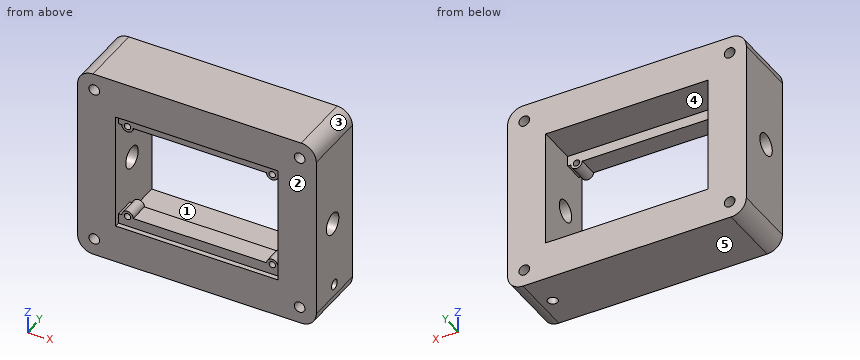
```python
from build123d import *

# Parameters (mm, degrees)
SKETCH1_W               = 94
SKETCH1_H               = 76
SKETCH1_R               = 1.25
BOSS_EXTRUDE1_DEPTH     = 9.8
SKETCH2_W               = 94
SKETCH2_H               = 76
SKETCH2_W_2             = 64
SKETCH2_H_2             = 46
BOSS_EXTRUDE3_DEPTH     = 15.2
SKETCH3_W               = 64
SKETCH3_H               = 46
CUT_EXTRUDE1_DEPTH      = 2
CUT_EXTRUDE2_DEPTH      = 105.427008001
CUT_EXTRUDE2_DEPTH_BACK = 105.427008001
SKETCH4_R               = 4.305
CUT_EXTRUDE3_DEPTH      = 66.406421703
CUT_EXTRUDE3_DEPTH_BACK = 66.406421703
SKETCH5_R               = 2.1
FILLET1_R               = 6
CUT_SWEEP_PROFILE_R     = 1.95


with BuildPart() as part:
    # Sketch1 → Boss-Extrude1 (new body)
    with BuildSketch(Plane(origin=(0, 0, 0), x_dir=(1, 0, 0), z_dir=(0, 1, 0))):
        Rectangle(SKETCH1_W, SKETCH1_H)
        with BuildLine():
            Line((-32, 19), (-30.75, 19))
            ThreePointArc((-30.75, 19), (-28.5, 16.75), (-26.25, 19))
            Line((-26.25, 19), (26.25, 19))
            ThreePointArc((26.25, 19), (28.5, 16.75), (30.75, 19))
            Line((30.75, 19), (32, 19))
            Line((32, 19), (32, -19))
            Line((32, -19), (30.75, -19))
            ThreePointArc((30.75, -19), (28.5, -16.75), (26.25, -19))
            Line((26.25, -19), (-26.25, -19))
            ThreePointArc((-26.25, -19), (-28.5, -16.75), (-30.75, -19))
            Line((-30.75, -19), (-32, -19))
            Line((-32, -19), (-32, 19))
        make_face(mode=Mode.SUBTRACT)
        with Locations(Location((-28.5, 19, 0), (0, 0, 270))):
            Circle(SKETCH1_R, mode=Mode.SUBTRACT)
        with Locations(Location((28.5, 19, 0), (0, 0, 270))):
            Circle(SKETCH1_R, mode=Mode.SUBTRACT)
        with Locations(Location((28.5, -19, 0), (0, 0, 270))):
            Circle(SKETCH1_R, mode=Mode.SUBTRACT)
        with Locations(Location((-28.5, -19, 0), (0, 0, 270))):
            Circle(SKETCH1_R, mode=Mode.SUBTRACT)
    extrude(amount=BOSS_EXTRUDE1_DEPTH)

    # Sketch2 → Boss-Extrude3 (add)
    with BuildSketch(Plane(origin=(0, 9.8, 0), x_dir=(1, 0, 0), z_dir=(0, 1, 0))):
        Rectangle(SKETCH2_W, SKETCH2_H)
        Rectangle(SKETCH2_W_2, SKETCH2_H_2, mode=Mode.SUBTRACT)
    extrude(amount=BOSS_EXTRUDE3_DEPTH)

    # Sketch3 → Cut-Extrude1 (cut)
    with BuildSketch(Plane.XZ):
        Rectangle(SKETCH3_W, SKETCH3_H)
    extrude(amount=-CUT_EXTRUDE1_DEPTH, mode=Mode.SUBTRACT)

    # Sketch4 → Cut-Extrude2 (cut, two sides: drawn at the far end of the back side and taken through both)
    with BuildSketch(Plane(origin=(47, 0, 0), x_dir=(0, 0, -1), z_dir=(1, 0, 0)).offset(-CUT_EXTRUDE2_DEPTH_BACK)):
        with Locations((1, 11.3)):
            Circle(SKETCH4_R)
    extrude(amount=CUT_EXTRUDE2_DEPTH + CUT_EXTRUDE2_DEPTH_BACK, mode=Mode.SUBTRACT)

    # Sketch5 → Cut-Extrude3 (cut, two sides: drawn at the far end of the back side and taken through both)
    with BuildSketch(Plane(origin=(0, 25, 0), x_dir=(1, 0, 0), z_dir=(0, 1, 0)).offset(-CUT_EXTRUDE3_DEPTH_BACK)):
        with Locations(Location((-40.44, 31.44, 0), (0, 0, 270))):
            Circle(SKETCH5_R)
        with Locations(Location((40.44, 31.44, 0), (0, 0, 270))):
            Circle(SKETCH5_R)
        with Locations(Location((40.44, -31.44, 0), (0, 0, 270))):
            Circle(SKETCH5_R)
        with Locations(Location((-40.44, -31.44, 0), (0, 0, 270))):
            Circle(SKETCH5_R)
    extrude(amount=CUT_EXTRUDE3_DEPTH + CUT_EXTRUDE3_DEPTH_BACK, mode=Mode.SUBTRACT)

    # Fillet1
    fillet1_edges = [part.edges().sort_by_distance(p)[0] for p in [
        (-47, 12.5, 38),
        (-47, 12.5, -38),
        (47, 12.5, -38),
        (47, 12.5, 38),
    ]]
    fillet(fillet1_edges, radius=FILLET1_R)

    # Cut-Sweep: sweep along a path in Sketch9
    with BuildLine(Plane(origin=(0, 12.5, 0), x_dir=(-1, 0, 0), z_dir=(0, -1, 0))) as cut_sweep_path:
        Line((-47, 27.34), (-40.44, 27.34))
        ThreePointArc((-40.44, 27.34), (-37.540862197, 28.540862197), (-36.34, 31.44))
        Line((-36.34, 31.44), (-36.34, 38))
    # Cut-Sweep profile (on start of the path) → Cut-Sweep (sweep, cut)
    with BuildSketch(Plane(origin=(47, 12.5, -27.34), x_dir=(0, 0, -1), z_dir=(-1, 0, 0))):
        Circle(CUT_SWEEP_PROFILE_R)
    sweep(path=cut_sweep_path.line, mode=Mode.SUBTRACT)


solid = part.part
```
Geometry: final body of the model. Coordinates: model frame, mm. Face numbers are marked on the shaded views. A direction names the side the tool comes from. Round coordinates to 2 decimals unless told otherwise and drop trailing zeros. Loops run counter-clockwise (first coordinate to the right, second up) from the corner with the lowest first, then second, coordinate; pieces in that order, holes last. Notation, with made-up numbers: (31, 81.25) -> (89, 81.25) arc R28 cw to (89, 108.25) -> close; hole circle Ø3 at (69.5, 80.5). An arc over 180 degrees is marked (long way). Write each question's results on one line, items separated by ' | '.
Item 1: Pull-direction query (X, two-part tool) for the marked faces 1, 2 and 3; classes: pulls with the +X half, pulls with the -X half, needs draft (parallel to the pull), parting line crosses it, or undercut.
Answers below:
face 1: undercut | face 2: needs draft | face 3: pulls with the +X half
Item 2: Cut plane C-C on x = 3. Return the cut outline in (y, z), and give its area (3 significant figures).
Answers below:
outline: (0, -38) -> (25, -38) -> (25, -23) -> (9.8, -23) -> (9.8, -19) -> (2, -19) -> (2, -23) -> (0, -23) -> close; (0, 23) -> (2, 23) -> (2, 19) -> (9.8, 19) -> (9.8, 23) -> (25, 23) -> (25, 38) -> (0, 38) -> close | area: 812 mm²
Item 3: Cut plane B-B on x = -28.5. Return the cut outline in (y, z), and give its area (4 significant figures).
Answers below:
outline: (0, -38) -> (25, -38) -> (25, -23) -> (9.8, -23) -> (9.8, -20.25) -> (2, -20.25) -> (2, -23) -> (0, -23) -> close; (0, 23) -> (2, 23) -> (2, 20.25) -> (9.8, 20.25) -> (9.8, 23) -> (25, 23) -> (25, 38) -> (0, 38) -> close; (2, -17.75) -> (9.8, -17.75) -> (9.8, -16.75) -> (2, -16.75) -> close; (2, 16.75) -> (9.8, 16.75) -> (9.8, 17.75) -> (2, 17.75) -> close | area: 808.5 mm²
Item 4: Set-up query: the marked faces 4 and 5. Return all of +Z, -Z, +X, -X, +Y, -Y with unobstructed straight access to the full face (end or side cutting, diameter ignored); none if empty.
Answers below:
face 4: +Y | face 5: -Z, +X, -X, +Y, -Y
Item 5: Pin query (flat end, axial travel): pin 1 Ø3 at (y, z) = (12.5, -27.34) entering from +X; pin 2 Ø4 at (x, z) = (28.5, 19) entering from +Y; pin 3 Ø6 at (x, z) = (-13.5, -14) entering from +Y; pin 4 Ø1.9 at (x, z) = (7.5, 21.5) entering from -Y. Return the tip coordinate at first contact, or that it passes through.
Answers below:
pin 1: stops at x = 38.15 | pin 2: stops at y = 9.8 | pin 3: passes through | pin 4: stops at y = 2
Item 6: Cut plane D-D on z = -1. Return the cut outline in (x, y) (3 decimals).
Answers below:
outline: (-47, 0) -> (-32, 0) -> (-32, 6.995) -> (-47, 6.995) -> close; (-47, 15.605) -> (-32, 15.605) -> (-32, 25) -> (-47, 25) -> close; (32, 0) -> (47, 0) -> (47, 6.995) -> (32, 6.995) -> close; (32, 15.605) -> (47, 15.605) -> (47, 25) -> (32, 25) -> close
Item 7: Line query: probe 1 along Z at (x, y) = (-28.5, 5); probe 2 along Z at (x, y) = (-4.5, 14.5); probe 3 along Z at (x, y) = (23, 6.5). Output: solid intervals per line, ascending. Write a range as [from, to].
Answers below:
probe 1: z = [-38, -20.25], [-17.75, -16.75], [16.75, 17.75], [20.25, 38] | probe 2: z = [-38, -23], [23, 38] | probe 3: z = [-38, -19], [19, 38]
Item 8: Cut plane A-A on z = 11. Return the cut outline in (x, y), and give its area (3 significant figures).
Answers below:
outline: (-47, 0) -> (-32, 0) -> (-32, 25) -> (-47, 25) -> close; (32, 0) -> (47, 0) -> (47, 25) -> (32, 25) -> close | area: 750 mm²
